Build history of the part. All positions in model axes, mm. A direction names the side the tool comes from. Round coordinates to 2 decimals unless told otherwise and drop trailing zeros. Loops run counter-clockwise (first coordinate to the right, second up) from the corner with the lowest first, then second, coordinate; pieces in that order, holes last. Notation, with made-up numbers: (-33.5, 50) - (-13.5, 50) arc R28 cw to (-13.5, 89) - close; hole circle Ø2 at (-29.75, 84.5). An arc over 180 degrees is marked (long way). Put each result on its own line as item: value. Start each with the question number.
from build123d import *

# Parameters (mm, degrees)
F2_R     = 21.8203360692
F3_DEPTH = 25.4
F4_R     = 32.3243741503
F4_R_2   = 21.5014025506
F5_DEPTH = 25.399999693
F6_R     = 3.81
F8_R     = 1.524


with BuildPart() as f3:
    # F2 (on face) → F3 (new body)
    with BuildSketch(Plane.XZ):
        with BuildLine():
            ThreePointArc((33.7495873612, -42.148321867), (27.0928879745, -22.0234599232), (9.7486972809, -9.8373709621))
            Line((9.7486972809, -9.8373709621), (9.7486972809, -16.04783535))
            Line((9.7486972809, -16.04783535), (-9.7486972809, -16.04783535))
            Line((-9.7486972809, -16.04783535), (-9.7486972809, -9.8373709621))
            ThreePointArc((-9.7486972809, -9.8373709621), (-20.1248619438, -69.2412098414), (33.7495873612, -42.148321867))
        make_face()
        with Locations((0, -42.148321867)):
            Circle(F2_R, mode=Mode.SUBTRACT)
        with BuildLine():
            Line((9.7486972809, -9.8373709621), (9.7486972809, 16.04783535))
            Line((9.7486972809, 16.04783535), (-9.7486972809, 16.04783535))
            Line((-9.7486972809, 16.04783535), (-9.7486972809, -9.8373709621))
            ThreePointArc((-9.7486972809, -9.8373709621), (0, -8.3987345058), (9.7486972809, -9.8373709621))
        make_face()
        with BuildLine():
            Line((9.7486972809, -16.04783535), (9.7486972809, -9.8373709621))
            ThreePointArc((9.7486972809, -9.8373709621), (0, -8.3987345058), (-9.7486972809, -9.8373709621))
            Line((-9.7486972809, -9.8373709621), (-9.7486972809, -16.04783535))
            Line((-9.7486972809, -16.04783535), (9.7486972809, -16.04783535))
        make_face()
    extrude(amount=-F3_DEPTH)

    # F4 (on Front) → F5 (join)
    with BuildSketch(Plane.XZ):
        with Locations((0, 41.2176400423)):
            Circle(F4_R)
        with Locations((0, 41.2176400423)):
            Circle(F4_R_2, mode=Mode.SUBTRACT)
    extrude(amount=-F5_DEPTH)

    # F6
    f6_edges = [f3.edges().sort_by_distance(p)[0] for p in [
        (-9.748697, 12.7, -9.837371),
        (-9.748697, 12.7, 10.398359),
        (9.748697, 12.7, 10.398359),
        (9.748697, 12.7, -9.837371),
    ]]
    fillet(f6_edges, radius=F6_R)

    # F8
    f8_edges = [f3.edges().sort_by_distance(p)[0] for p in [
        (0, 0, -75.897909),
        (-12.183319, 12.7, -10.674501),
        (12.183319, 12.7, -10.674501),
        (0, 25.4, -75.897909),
        (10.415746, 0, -9.275004),
        (9.748697, 12.7, -7.121413),
        (10.415746, 25.4, -9.275004),
        (-10.415746, 0, -9.275004),
        (-9.748697, 12.7, -7.121413),
        (-10.415746, 25.4, -9.275004),
        (10.399348, 25.4, 9.853003),
        (12.129071, 12.7, 11.25515),
        (9.748697, 12.7, 7.72354),
        (10.399348, 0, 9.853003),
        (0, 0, 73.542014),
        (-12.129071, 12.7, 11.25515),
        (0, 25.4, 73.542014),
        (-10.399348, 25.4, 9.853003),
        (-9.748697, 12.7, 7.72354),
        (-10.399348, 0, 9.853003),
    ]]
    fillet(f8_edges, radius=F8_R)


solid = f3.part
1) Drop flat-ended pins along their axis: pin 1 Ø6 at (y, z) = (4, -30) entering from +X; pin 2 Ø1 at (y, z) = (4, 55.5) entering from -X; pin 3 Ø4.5 at (y, z) = (10, -2.5) entering from +X. Give the stop position or say it passes through.
2) Slice it at B-B, the plane z = 0. Write the cut outline in (x, y).
3) Drill centre lines: line 1 (Z direction, x = 0, y = 17); line 2 (Z direction, x = -17.5, y = 6); line 3 (Z direction, x = -16, y = 3.75) (3 decimals). Where is each one in solid material? Low to high. Write a range as [from, to].
4) Pull direction Z, two halves, no side cores. Call faces 4 (the face through (0, 0, 0)), 5 (the face through (9.749, 13, 0)): pulls with the +Z half, pulls with the -Z half, needs draft (parallel to the pull), parting line crosses it, or undercut.
5) Slice it at A-A, the plane x = 0. State how many separate pieces and enclosed holes the cut face has, and give its area (3 significant figures).
6) Which spindle directions (+Z, -Z, +X, -X, +Y, -Y) get a long thin tool onto all of the face, cutting with end or side? Do faces 1 (the face through (-10.42, 12.54, 9.88)), 2 (the face through (-4.73, 12.52, -63.45)), 3 (the face through (10.434, 12.856, -9.301)). Say none if no direction does.
7) Slice it at C-C, the plane y = 10.5. Write the cut outline in (x, z), and give its area (3 significant figures).
Taken from the geometry:
1. pin 1: stops at x = 32.49
1. pin 2: stops at x = -29.24
1. pin 3: stops at x = 9.75
2. outline: (-9.75, 1.52) arc R1.52 ccw to (-8.22, 0) - (8.22, 0) arc R1.52 ccw to (9.75, 1.52) - (9.75, 23.88) arc R1.52 ccw to (8.22, 25.4) - (-8.22, 25.4) arc R1.52 ccw to (-9.75, 23.88) - close
3. line 1: z = [-75.9, -63.97], [-20.33, 19.72], [62.72, 73.54]
3. line 2: z = [-71.01, -55.18], [-29.11, -13.29], [14.04, 28.73], [53.71, 68.4]
3. line 3: z = [-71.864, -56.985], [-27.312, -12.432], [13.131, 26.854], [55.581, 69.304]
4. face 4: needs draft
4. face 5: undercut
5. separate pieces: 3
5. enclosed holes: 0
5. area: 1,590 mm2
6. face 1: -X, +Y, -Y
6. face 2: +Y, -Y
6. face 3: +X, +Y, -Y
7. outline: (-12.18, -10.67) arc R33.75 ccw (long way) to (12.18, -10.67) arc R3.81 cw to (9.75, -7.12) - (9.75, 7.72) arc R3.81 cw to (12.13, 11.26) arc R32.32 ccw (long way) to (-12.13, 11.26) arc R3.81 cw to (-9.75, 7.72) - (-9.75, -7.12) arc R3.81 cw to start; hole circle Ø43.64 at (0, -42.15); hole circle Ø43 at (0, 41.22)
7. area: 4,270 mm2
